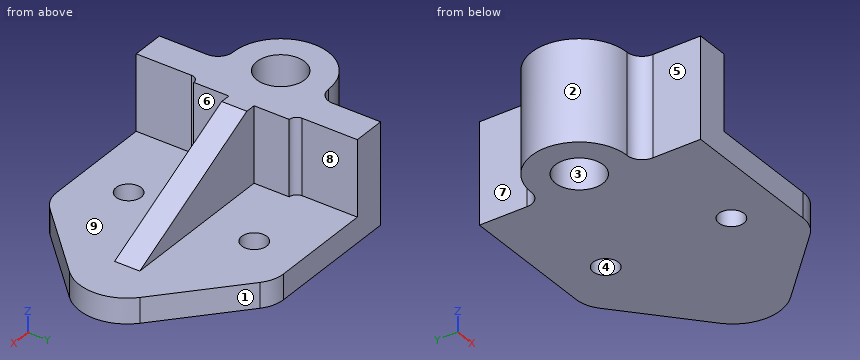
Autodesk Fusion 360 part; units mm, degrees
sketch "Sketch1" plane through (0, 0, 0) normal (0, 0, 1) x (1, 0, 0)
  line L0 (16.3701, -44) -> (-33.5, -44)
  line L1 (-33.5, 44) -> (12.6952, 44)
  line L2 (-26.5, 5) -> (-30.5, 5) construction
  line L3 (-30.5, -5) -> (-26.5, -5) construction
  circle A0 centre (-2.5, 25) radius 5
  circle A1 centre (-2.5, -25) radius 5
  line L4 (46.935, 13.435) -> (46.9571, 13.4571)
  line L5 (46.935, -13.435) -> (16.3701, -44)
  line L6 (46.9571, 13.4571) -> (12.6952, 44)
  line L7 (-33.5, 44) -> (-46.5, 44)
  line L8 (-46.5, -44) -> (-33.5, -44)
  circle A2 centre (-52.5, 0) radius 9.5
  arc A3 (-52.5, 19) -> (-46.5, 25) centre (-52.5, 25) ccw
  arc A4 (-46.5, -25) -> (-52.5, -19) centre (-52.5, -25) ccw
  line L9 (-46.5, 25) -> (-46.5, 44) construction
  line L10 (-46.5, 44) -> (-46.5, 25)
  arc A5 (-52.5, 19) -> (-52.5, -19) centre (-52.5, 0) ccw
  line L11 (-46.5, -44) -> (-46.5, -25) construction
  line L12 (-46.5, -25) -> (-46.5, -44)
  line L13 (-33.5, -44) -> (-26.5, -44) construction
  arc A6 (-30.5, -19) -> (-33.5, -22) centre (-30.5, -22) ccw
  arc A7 (-33.5, 22) -> (-30.5, 19) centre (-30.5, 22) ccw
  line L14 (-33.5, -22) -> (-33.5, -44) construction
  line L15 (-33.5, 44) -> (-33.5, 22) construction
  line L16 (-33.5, 22) -> (-33.5, 44)
  line L17 (-33.5, 22) -> (-33.5, 44)
  line L18 (-33.5, -44) -> (-33.5, -22)
  line L19 (-33.5, -44) -> (-33.5, -22)
  arc A8 (46.935, -13.435) -> (46.1432, 14.1827) centre (33.5, 0) ccw
  line L20 (-30.5, -19) -> (-30.5, -5)
  line L21 (-30.5, 5) -> (-30.5, 19)
  line L22 (-30.5, -5) -> (-26.5, -5)
  line L23 (-26.5, -5) -> (-26.5, 5)
  line L24 (-26.5, 5) -> (-30.5, 5)
  dimension "d2" = 88
  dimension "d4" = 10
  dimension "d5" = 39
  dimension "d8" = 10
  dimension "d9" = 10
  dimension "d10" = 38
  dimension "d13" = 13
  dimension "d17" = 19
  dimension "d18" = 38
  dimension "d20" = 12
  dimension "d21" = 12
  dimension "d22" = 7
  dimension "d25" = 6
  dimension "d26" = 6
  dimension "d27" = 4
extrude "Extrude1" add sketch "Sketch1" along normal blind 40 contours L7 L8 A3 A4 L10 A5 L12 A6 A7 L16 L17 L18 L19 L20 L21 L22 L23 L24
extrude "Extrude2" add sketch "Sketch1" along normal blind 10 contours L0 L1 L5 L6 A6 A7 L16 L17 L18 L19 A8 L20 L21 L22 L23 L24
sketch "Sketch2" plane through (0, 0, 0) normal (0, 1, 0) x (1, 0, 0)
  line L0 (-26.5, -40) -> (-26.5, -10)
  line L1 (-26.5, -10) -> (33.5, -10)
  line L2 (33.5, -10) -> (-26.5, -40)
  dimension "d32" = 60
extrude "Extrude3" add sketch "Sketch2" along normal mid plane 10
fillet "Fillet1" radius 13 1 edges at (16.3701, -44, 5)
fillet "Fillet2" radius 13 1 edges at (12.6952, 44, 5)
equation "d5 = ( ( 88 - 10 ) / 2 ) * 1 mm"
equation "d10 = ( 19 * 2 ) * 1 mm"
Design review of the part built by this model. Coordinates are the model's own, in mm. Face numbers are marked on the shaded views. A direction names the side the tool comes from. Coordinates: 2 decimals unless noted, no trailing zeros. Order: outer loops, then holes, each group sorted by start corner. A loop starts at its lowest first (then second) coordinate and runs counter-clockwise, first axis right, second up. Notation, with made-up numbers: (42, -19.5) - (85, -19.5) arc R29 cw to (85, 10.5) - close; hole circle Ø7 at (33.5, 23.25). An arc over 180 degrees is marked (long way). One line per question, with ' | ' between items.
Q1. Consider section A-A, the plane x = -2.5. Give the boundary of the cut face in (y, z).
Answer key:
outline: (-44, 0) - (-30, 0) - (-30, 10) - (-44, 10) - close; (-20, 0) - (20, 0) - (20, 10) - (5, 10) - (5, 28) - (-5, 28) - (-5, 10) - (-20, 10) - close; (30, 0) - (44, 0) - (44, 10) - (30, 10) - close
Q2. The part is to be moulded in two halves that separate along X. For the marked faces 1, 2, 3 and 4, say which applies: +X half, -X half, draft (parallel to the pull), parting line (faces both ways), or undercut.
Answer key:
face 1: +X half | face 2: -X half | face 3: undercut | face 4: undercut
Q3. To check wall thickness, follow line 1 along Y through (x, z) = (-2, 7.5); line 2 along Y through (x, z) = (-52.5, 22); line 3 along Z through (x, y) = (-0.5, -36). State the ranges of each line that lie inside material, in increasing order.
Answer key:
line 1: y = -44 to -29.97, -20.03 to 20.03, 29.97 to 44 | line 2: y = -19 to -9.5, 9.5 to 19 | line 3: z = 0 to 10
Q4. Consider section D-D, the plane x = -16. Give the boundary of the cut face in (y, z).
Answer key:
outline: (-44, 0) - (44, 0) - (44, 10) - (5, 10) - (5, 34.75) - (-5, 34.75) - (-5, 10) - (-44, 10) - close
Q5. For the marked faces 5, 6, 7, 8 and 9, list the 3-axis set-ups (+Z, -Z, +X, -X, +Y, -Y) from which the entire face can be reached by the end or side of a thin tool; tool diameter is ignored.
Answer key:
face 5: +Z, -Z, -X, -Y | face 6: +Z, +X, -Y | face 7: +Z, -Z, -X, +Y | face 8: +Z, +X, +Y | face 9: +Z, +X
Q6. Consider section B-B, the plane z = 24.5. Give the boundary of the cut face in (x, y).
Answer key:
outline: (-52.5, -19) arc R6 cw to (-46.5, -25) - (-46.5, -44) - (-33.5, -44) - (-33.5, -22) arc R3 cw to (-30.5, -19) - (-30.5, -5) - (4.5, -5) - (4.5, 5) - (-30.5, 5) - (-30.5, 19) arc R3 cw to (-33.5, 22) - (-33.5, 44) - (-46.5, 44) - (-46.5, 25) arc R6 cw to (-52.5, 19) arc R19 ccw to start; hole circle Ø19 at (-52.5, 0)
Q7. Clearance check with flat-ended pins moving along their axes: pin 1 Ø2 at (y, z) = (18, 35.5) entering from +X; pin 2 Ø15 at (x, z) = (16, 18.5) entering from -Y; pin 3 Ø9 at (x, y) = (-2.5, -25) entering from -Z; pin 4 Ø10 at (x, y) = (-0.5, -21.5) entering from +Z. State where each tip first meets the part, or that it passes through.
Answer key:
pin 1: stops at x = -30.5 | pin 2: stops at y = -5 | pin 3: passes through | pin 4: stops at z = 10
Q8. Consider section C-C, the plane y = 27. Give the boundary of the cut face in (x, z), then the cut area to 3 significant figures.
Answer key:
outline: (-46.5, 0) - (-7.08, 0) - (-7.08, 10) - (-33.5, 10) - (-33.5, 40) - (-46.5, 40) - close; (2.08, 0) - (31.77, 0) - (31.77, 10) - (2.08, 10) - close | area: 1,080 mm2
